The listing builds one solid part. Answer for the finished solid, in the listing's coordinates (mm). A direction names the side the tool comes from. Coordinates: 2 decimals unless noted, no trailing zeros. Loops run counter-clockwise (first coordinate to the right, second up) from the corner with the lowest first, then second, coordinate; pieces in that order, holes last. Notation, with made-up numbers: (60, 23.5) - (89, 23.5) arc R15 cw to (89, 43.5) - close; hole circle Ø8 at (39, 85.5). An arc over 180 degrees is marked (long way). Put each result on its own line as item: value.
```python
from build123d import *

# Parameters (mm, degrees)
SKETCH_1_W      = 22
SKETCH_1_H      = 28
SKETCH_1_R      = 1.3
SKETCH_1_R_2    = 0.5
EXTRUDE_1_DEPTH = 1.6
SKETCH_2_W      = 5.2
SKETCH_2_H      = 4.3
EXTRUDE_2_DEPTH = 0.91


with BuildPart() as part:
    # 草图1 → 凸台-拉伸1 (new body)
    with BuildSketch(Plane.XY):
        Rectangle(SKETCH_1_W, SKETCH_1_H)
        with Locations((-9, -1)):
            Circle(SKETCH_1_R, mode=Mode.SUBTRACT)
        with Locations((-9, -12)):
            Circle(SKETCH_1_R, mode=Mode.SUBTRACT)
        with Locations(Location((9, -12, 0), (0, 0, 180))):
            Circle(SKETCH_1_R, mode=Mode.SUBTRACT)
        with Locations(Location((9, -1, 0), (0, 0, 180))):
            Circle(SKETCH_1_R, mode=Mode.SUBTRACT)
        with Locations((-8.89, 10.8)):
            Circle(SKETCH_1_R_2, mode=Mode.SUBTRACT)
        with Locations((-6.35, 10.8)):
            Circle(SKETCH_1_R_2, mode=Mode.SUBTRACT)
        with Locations((-3.81, 10.8)):
            Circle(SKETCH_1_R_2, mode=Mode.SUBTRACT)
        with Locations((-1.27, 10.8)):
            Circle(SKETCH_1_R_2, mode=Mode.SUBTRACT)
        with Locations((1.27, 10.8)):
            Circle(SKETCH_1_R_2, mode=Mode.SUBTRACT)
        with Locations((3.81, 10.8)):
            Circle(SKETCH_1_R_2, mode=Mode.SUBTRACT)
        with Locations((6.35, 10.8)):
            Circle(SKETCH_1_R_2, mode=Mode.SUBTRACT)
        with Locations((8.89, 10.8)):
            Circle(SKETCH_1_R_2, mode=Mode.SUBTRACT)
        with Locations((-6.35, 8.26)):
            Circle(SKETCH_1_R_2, mode=Mode.SUBTRACT)
        with Locations((-3.81, 8.26)):
            Circle(SKETCH_1_R_2, mode=Mode.SUBTRACT)
        with Locations((-1.27, 8.26)):
            Circle(SKETCH_1_R_2, mode=Mode.SUBTRACT)
        with Locations((1.27, 8.26)):
            Circle(SKETCH_1_R_2, mode=Mode.SUBTRACT)
        with Locations((3.81, 8.26)):
            Circle(SKETCH_1_R_2, mode=Mode.SUBTRACT)
        with Locations((6.35, 8.26)):
            Circle(SKETCH_1_R_2, mode=Mode.SUBTRACT)
        with Locations((8.89, 8.26)):
            Circle(SKETCH_1_R_2, mode=Mode.SUBTRACT)
        with Locations((-8.89, 8.26)):
            Circle(SKETCH_1_R_2, mode=Mode.SUBTRACT)
    extrude(amount=EXTRUDE_1_DEPTH)

    # 草图2 → 凸台-拉伸2 (add)
    with BuildSketch(Plane.XY.offset(1.6)):
        with Locations((0, -6.5)):
            Rectangle(SKETCH_2_W, SKETCH_2_H)
    extrude(amount=EXTRUDE_2_DEPTH)


solid = part.part
```
1) The part is cut by section B-B (z = 0.65). State how many separate pieces and enclosed holes the cut face has, and give its area (3 significant figures).
Found:
separate pieces: 1
enclosed holes: 20
area: 582 mm^2
2) Each of these flat-tipped pins is pushed along its axis until it touches: pin 1 (2 mm diameter, centred on x = -9, y = -1, fed in from -Z); pin 2 (1.5 mm diameter, centred on x = 7, y = -8, fed in from +Z); pin 3 (0.7 mm diameter, centred on x = -1, z = 2, fed in from -Y); pin 4 (0.7 mm diameter, centred on y = -5.5, z = 2.5, fed in from -X). Where does it stop, or does it pass through?
Found:
pin 1: passes through
pin 2: stops at z = 1.6
pin 3: stops at y = -8.65
pin 4: stops at x = -2.6
3) The part is cut by section D-D (x = -9). Give the vertices of the cut face in (y, z).
Found:
outline: (-14, 0) - (-13.3, 0) - (-13.3, 1.6) - (-14, 1.6) - close; (-10.7, 0) - (-2.3, 0) - (-2.3, 1.6) - (-10.7, 1.6) - close; (0.3, 0) - (7.77, 0) - (7.77, 1.6) - (0.3, 1.6) - close; (8.75, 0) - (10.31, 0) - (10.31, 1.6) - (8.75, 1.6) - close; (11.29, 0) - (14, 0) - (14, 1.6) - (11.29, 1.6) - close
4) For a pull along X with two mould halves and no side action, classify faces 4 (the face through (-5.888, 10.608, 0.789)), 5 (the face through (-2.6, -7, 2)), 6 (the face through (0, -6, 2.51)) as pulls with the +X half, pulls with the -X half, needs draft (parallel to the pull), parting line crosses it, or undercut.
Found:
face 4: undercut
face 5: pulls with the -X half
face 6: needs draft
5) Straight lines are drawn through the part: L1, parallel to Y at x = -8.89, z = 0.8; L2, parallel to Y at x = -3.81, z = 0.4; L3, parallel to Y at x = -9, z = 1.35. For each, find the intervals that lie inside material, in ascending order. Write a range as [from, to].
Found:
L1: y = [-14, -13.3], [-10.7, -2.3], [0.3, 7.76], [8.76, 10.3], [11.3, 14]
L2: y = [-14, 7.76], [8.76, 10.3], [11.3, 14]
L3: y = [-14, -13.3], [-10.7, -2.3], [0.3, 7.77], [8.75, 10.31], [11.29, 14]
6) The part is cut by section A-A (x = -1.27). Give the vertices of the cut face in (y, z).
Found:
outline: (-14, 0) - (7.76, 0) - (7.76, 1.6) - (-4.35, 1.6) - (-4.35, 2.51) - (-8.65, 2.51) - (-8.65, 1.6) - (-14, 1.6) - close; (8.76, 0) - (10.3, 0) - (10.3, 1.6) - (8.76, 1.6) - close; (11.3, 0) - (14, 0) - (14, 1.6) - (11.3, 1.6) - close
7) The part is cut by section C-C (y = -5.25). Give the vertices of the cut face in (x, z), and give its area (3 significant figures).
Found:
outline: (-11, 0) - (11, 0) - (11, 1.6) - (2.6, 1.6) - (2.6, 2.51) - (-2.6, 2.51) - (-2.6, 1.6) - (-11, 1.6) - close
area: 39.9 mm^2
8) For faces 1 (the face through (2.6, -7, 2)), 2 (the face through (7.76, -1.39, 0.79)), 3 (the face through (0, -4.35, 2)), determine the directions among +Z, -Z, +X, -X, +Y, -Y from which every point of the face is accessible in a straight line to the end or side of a thin tool.
Found:
face 1: +Z, +X, +Y, -Y
face 2: +Z, -Z
face 3: +Z, +X, -X, +Y
